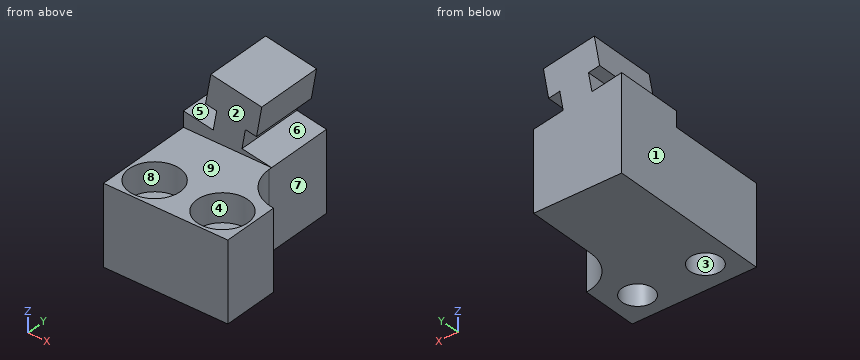
Autodesk Inventor part; units mm, degrees
ref_plane "YZ Plane" through (0, 0, 0) normal (1, 0, 0) x (0, 1, 0)
ref_plane "XZ Plane" through (0, 0, 0) normal (0, 1, 0) x (-1, 0, 0)
ref_plane "XY Plane" through (0, 0, 0) normal (0, 0, 1) x (1, 0, 0)
sketch "Sketch5" plane through (0, 0, 0) normal (0, 0, 1) x (1, 0, 0)
  line L0 (0, 0) -> (-15.6, 0)
  line L1 (-15.6, 0) -> (-15.6, -29.5)
  line L2 (-15.6, -29.5) -> (6.4, -29.5)
  line L3 (6.4, -29.5) -> (6.4, -19.5)
  line L4 (0, 0) -> (0, -12.526)
  line L5 (0, -12.526) -> (0, -19.5)
  line L6 (0, -19.5) -> (6.4, -19.5)
  dimension "d111" = 15.6
  dimension "d112" = 29.5
  dimension "d113" = 22
  dimension "d114" = 10
  dimension "d116" = 12.526
extrude "Extrusion2" add sketch "Sketch5" along normal blind 14
sketch "Skizze14" plane through (0, 0, 14) normal (0, 0, 1) x (1, 0, 0)
  line L0 (-15.6, -29.5) -> (6.4, -29.5)
  line L1 (-15.6, 0) -> (-15.6, -29.5)
  circle A0 centre (-10.6, -24.5) radius 4.5
  circle A1 centre (1.4, -24.5) radius 4.5
  circle A2 centre (-10.6, -24.5) radius 2.75
  circle A3 centre (1.4, -24.5) radius 2.75
  point P0 (0, 0)
  dimension "d117" = 5
  dimension "d118" = 5
  dimension "d119" = 12
  dimension "d120" = 5
  dimension "d121" = 9
  dimension "d122" = 9
  dimension "d123" = 5.5
  dimension "d124" = 5.5
extrude "Extrusion9" cut sketch "Skizze14" against normal blind 5 contours A0 | A1 | A2 | A3
sketch "Skizze16" plane through (0, 0, 14) normal (0, 0, 1) x (1, 0, 0)
  circle A0 centre (-10.6, -24.5) radius 2.75
  circle A1 centre (1.4, -24.5) radius 2.75
  line L0 (-15.6, 0) -> (-15.6, -29.5)
  line L1 (-15.6, -29.5) -> (6.4, -29.5)
  line L2 (6.4, -29.5) -> (6.4, -19.5)
  point P0 (0, 0)
  dimension "d127" = 5
  dimension "d128" = 5
  dimension "d129" = 5
  dimension "d130" = 5
  dimension "d131" = 5.5
  dimension "d132" = 5.5
extrude "Extrusion10" cut sketch "Skizze16" against normal blind 15
fillet "Rundung3" radius 7 1 edges at (0, -19.5, 7)
sketch "Skizze17" plane through (-15.6, 0, 0) normal (0, 1, 0) x (1, 0, 0)
  line L0 (0, -14) -> (22, -14)
  line L1 (0, -14) -> (0, -16.751)
  line L2 (0, -16.751) -> (5.264, -15.8228)
  line L3 (5.8718, -19.2696) -> (3.9022, -19.6169)
  line L4 (3.9022, -19.6169) -> (4.8399, -24.9349)
  line L5 (4.8399, -24.9349) -> (13.8508, -23.346)
  line L6 (10.3562, -14.9105) -> (15.6, -14)
  line L7 (5.264, -15.8228) -> (5.8718, -19.2696)
  line L8 (13.8508, -23.346) -> (12.9251, -18.0147)
  line L9 (12.9251, -18.0147) -> (10.9546, -18.3569)
  line L10 (10.9546, -18.3569) -> (10.3562, -14.9105)
  point P0 (15.6, 0)
  dimension "d136" = 2.751
  dimension "d137" = 80
  dimension "d141" = 3.5
  dimension "d143" = 2
  dimension "d144" = 5.4
  dimension "d145" = 9.15
  dimension "d147" = 2
extrude "Extrusion11" add sketch "Skizze17" against normal blind 12
equation "\"l1\" = 8"
properties part number "Finray_9_Kerbe_10deg_anschluss_erweitert_9_75 Nut"
Input: part model. Units: mm. Frame: model coordinates. Face numbers are marked on the shaded views. A direction names the side the tool comes from. Coordinates: 2 decimals unless noted, no trailing zeros. Order: outer loops, then holes, each group sorted by start corner. A loop starts at its lowest first (then second) coordinate and runs counter-clockwise, first axis right, second up. Notation, with made-up numbers: (13, 84.5) - (29, 84.5) arc R19 ccw to (29, 88.5) - close; hole circle Ø6 at (75, -0.75). An arc over 180 degrees is marked (long way). Return JSON: item names as keys, results as strings.
Q1. Ray query, probe 1 along X at (y, z) = (-27.25, 13); probe 2 along Z at (x, y) = (0.25, -19.5); probe 3 along Y at (x, z) = (-10.6, 3.5). Return the intervals inside material, ascending.
The answers:
{"probe 1": "x = -15.6 to -14.16, -7.04 to -2.16, 4.96 to 6.4", "probe 2": "z = 0 to 14", "probe 3": "y = -29.5 to -27.25, -21.75 to 0"}
Q2. Cut plane D-D (y = -8.5). Return loops of the section in (x, z), then the cut area to 3 significant figures.
The answers:
{"outline": "(-15.6, 0) - (0, 0) - (0, 14) - (-5.24, 14.91) - (-4.65, 18.36) - (-2.67, 18.01) - (-1.75, 23.35) - (-10.76, 24.93) - (-11.7, 19.62) - (-9.73, 19.27) - (-10.34, 15.82) - (-15.6, 16.75) - close", "area": "307 mm2"}
Q3. Cut plane A-A (y = -24.5). Return loops of the section in (x, z).
The answers:
{"outline": "(-15.6, 0) - (-13.35, 0) - (-13.35, 9) - (-15.1, 9) - (-15.1, 14) - (-15.6, 14) - close; (-7.85, 0) - (-1.35, 0) - (-1.35, 9) - (-3.1, 9) - (-3.1, 14) - (-6.1, 14) - (-6.1, 9) - (-7.85, 9) - close; (4.15, 0) - (6.4, 0) - (6.4, 14) - (5.9, 14) - (5.9, 9) - (4.15, 9) - close"}
Q4. Cut plane C-C (x = -9.25). Return loops of the section in (y, z).
The answers:
{"outline": "(-29.5, 0) - (-26.9, 0) - (-26.9, 9) - (-28.79, 9) - (-28.79, 14) - (-29.5, 14) - close; (-22.1, 0) - (0, 0) - (0, 24.67) - (-12, 24.67) - (-12, 14) - (-20.21, 14) - (-20.21, 9) - (-22.1, 9) - close"}
Q5. Draft query along X for the marked faces 1, 2, 3 and 4. Return one class per face: +X half, -X half, draft (parallel to the pull), parting line (faces both ways), or undercut.
The answers:
{"face 1": "-X half", "face 2": "draft", "face 3": "undercut", "face 4": "undercut"}
Q6. First-contact query: pin 1 (7 mm diameter, centred on x = 0, y = -26.5, fed in from +Z); pin 2 (2.5 mm diameter, centred on x = -8.5, y = -22.5, fed in from +Z); pin 3 (14 mm diameter, centred on y = -3.5, z = 6.5, fed in from +X); pin 4 (9 mm diameter, centred on x = 1.4, y = -24.5, fed in from -Z). Flat tips, straight axial feed; report the tip coordinate or a pass-through.
The answers:
{"pin 1": "stops at z = 14", "pin 2": "stops at z = 9", "pin 3": "stops at x = 0", "pin 4": "stops at z = 0"}
Q7. Cut plane B-B (z = 7.5). Return loops of the section in (x, y).
The answers:
{"outline": "(-15.6, -29.5) - (6.4, -29.5) - (6.4, -19.5) arc R7 cw to (0, -12.53) - (0, 0) - (-15.6, 0) - close; hole circle Ø5.5 at (-10.6, -24.5); hole circle Ø5.5 at (1.4, -24.5)"}
Q8. Access query for the marked faces 5, 6, 7, 8 and 9. Directions: +Z, -Z, +X, -X, +Y, -Y. A direction counts if a zero-diameter tool reaches every point of the face in a straight line with its end or side. Return the directions, or none.
The answers:
{"face 5": "+Y, -Y", "face 6": "+X, +Y, -Y", "face 7": "+Z, -Z, +X, +Y", "face 8": "+Z", "face 9": "+Z, +X, -X, -Y"}
